Verification items for the finished model (mm, model axes). Face numbers are marked on the shaded views. A direction names the side the tool comes from. Round coordinates to 2 decimals unless told otherwise and drop trailing zeros. Order: outer loops, then holes, each group sorted by start corner. A loop starts at its lowest first (then second) coordinate and runs counter-clockwise, first axis right, second up. Notation, with made-up numbers: (80.5, 69.5) -> (88.5, 69.5) arc R37 ccw to (88.5, 108.5) -> close; hole circle Ø6 at (80.5, 89). An arc over 180 degrees is marked (long way). Return JSON: item names as keys, results as strings. Group by question number.
1) Scan lines: L1, parallel to X at y = -12, z = 10.5; L2, parallel to Y at x = 15, z = -2; L3, parallel to Z at x = 5, y = -8.5. Record each from-to range of solid material in increasing order.
2) Section check A-A on y = 0. Enter the section's corners in (x, z).
3) Depth check by flat-ended pin: pin 1 (10 mm diameter, centred on y = -10, z = 12.5, fed in from +X); pin 2 (5 mm diameter, centred on x = 39.5, y = 2, fed in from +Z); pin 3 (6 mm diameter, centred on x = 60, y = 6, fed in from -Z). Enter the tip coordinate at first touch or a pass-through.
4) Section check C-C on x = 42. Enter the section's corners in (y, z).
5) Tool access check on the marked faces 1 and 2. Record the directions out of +Z, -Z, +X, -X, +Y, -Y that give a thin tool (end or side, any length) a straight path to the whole face; none if there is none.
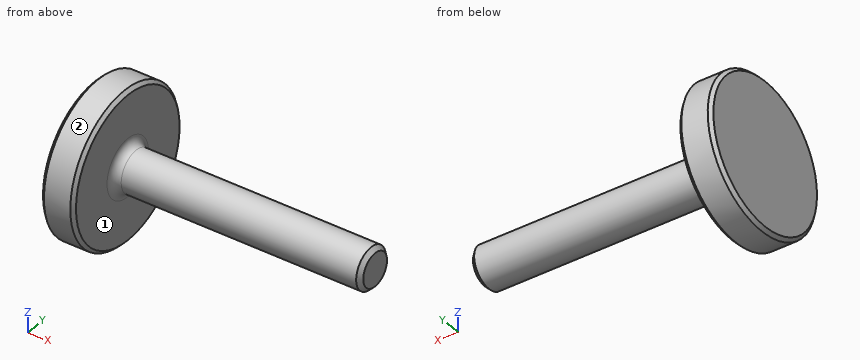
```python
from build123d import *

# Parameters (mm, degrees)
FILLET2_R     = 2
SKETCH1_R     = 0.5
NOTHING_DEPTH = 2


with BuildPart() as part:
    # BodySke → Base-Revolve (revolve)
    with BuildSketch(Plane.XY, mode=Mode.PRIVATE) as base_revolve_sk:
        Polygon((67, 5), (68, 4), (68, 0), (0, 0), (0, 17.45), (0.8, 18.25), (7.2, 18.25), (8, 17.45), (8, 5), align=None)
    revolve(base_revolve_sk.sketch.rotate(Axis((-11.400788802, 0, 0), (1, 0, 0)), 90), axis=Axis((-11.400788802, 0, 0), (1, 0, 0)))

    # Fillet2
    fillet2_edges = [part.edges().sort_by_distance(p)[0] for p in [
        (8, 0, -5),
    ]]
    fillet(fillet2_edges, radius=FILLET2_R)

    # Sketch1 → Nothing (add)
    with BuildSketch(Plane(origin=(68, 0, 0), x_dir=(0, 0, -1), z_dir=(1, 0, 0))):
        Circle(SKETCH1_R)
    extrude(amount=-NOTHING_DEPTH)


solid = part.part
```
Check result:
{
 "1": {"L1": "0 to 8", "L2": "-4.58 to 4.58", "L3": "-16.15 to 16.15"},
 "2": {"outline": "(0, -17.45) -> (0.8, -18.25) -> (7.2, -18.25) -> (8, -17.45) -> (8, -7) arc R2 cw to (10, -5) -> (67, -5) -> (68, -4) -> (68, 4) -> (67, 5) -> (10, 5) arc R2 cw to (8, 7) -> (8, 17.45) -> (7.2, 18.25) -> (0.8, 18.25) -> (0, 17.45) -> close"},
 "3": {"pin 1": "x = 8", "pin 2": "z = 5", "pin 3": "z = -4"},
 "4": {"outline": "circle Ø10 at (0, 0)"},
 "5": {"face 1": "+X", "face 2": "+X, -X"}
}
